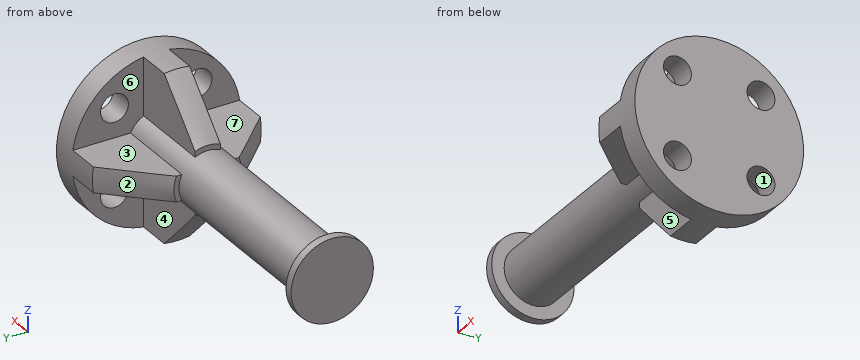
Solid Edge part; units mm, degrees
sketch "Sketch1" plane through (0, 0, 0) normal (-1, 0, 0) x (0, -1, 0)
  circle A0 centre (0, 0) radius 10
extrude "Protrusion1" add sketch "Sketch1" along normal blind 3
sketch "Sketch2" plane through (-3, 0, 0) normal (-1, 0, 0) x (0, -1, 0)
  circle A0 centre (0, 0) radius 3.4
extrude "Protrusion2" add sketch "Sketch2" along normal blind 34.2
sketch "Sketch3" plane through (-3, 0, 0) normal (-1, 0, 0) x (0, -1, 0)
  line L0 (3.0512, 1.5) -> (9.8869, 1.5)
  arc A0 (9.8869, 1.5) -> (9.8869, -1.5) centre (0, 0) cw
  line L1 (3.0512, -1.5) -> (9.8869, -1.5)
  line L2 (3.0512, 1.5) -> (3.0512, -1.5)
  line L3 (1.5, 3.0512) -> (1.5, 9.8869)
  arc A1 (-1.5, 9.8869) -> (1.5, 9.8869) centre (0, 0) cw
  line L4 (-1.5, 3.0512) -> (-1.5, 9.8869)
  line L5 (-1.5, 3.0512) -> (1.5, 3.0512)
  line L6 (-3.0512, 1.5) -> (-9.8869, 1.5)
  arc A2 (-9.8869, 1.5) -> (-9.8869, -1.5) centre (0, 0) ccw
  line L7 (-9.8869, -1.5) -> (-3.0512, -1.5)
  line L8 (-3.0512, -1.5) -> (-3.0512, 1.5)
  line L9 (-1.5, -3.0512) -> (-1.5, -9.8869)
  arc A3 (-1.5, -9.8869) -> (1.5, -9.8869) centre (0, 0) ccw
  line L10 (1.5, -9.8869) -> (1.5, -3.0512)
  line L11 (1.5, -3.0512) -> (-1.5, -3.0512)
extrude "Protrusion3" add sketch "Sketch3" along normal blind 10
chamfer "Chamfer1" distance 6 angle 45 4 edges at (-13, -10, 0) (-13, 0, 10) (-13, 10, 0) (-13, 0, -10)
sketch "Sketch4" plane through (-3, 5.9983, -5.9983) normal (-1, 0, 0) x (0, -1, 0)
  circle A0 centre (1.0486, 1.0486) radius 1.65
  circle A1 centre (10.9481, 1.0486) radius 1.65
  circle A2 centre (10.9481, 10.9481) radius 1.65
  circle A3 centre (1.0486, 10.9481) radius 1.65
extrude "Cutout1" cut sketch "Sketch4" against normal up to next
sketch "Sketch5" plane through (-37.2, 0, 0) normal (-1, 0, 0) x (0, -1, 0)
  circle A0 centre (0, 0) radius 4.875
extrude "Protrusion4" add sketch "Sketch5" against normal blind 1
Read the model definition and answer for the solid it produces. Units are mm, in the model's axes. Face numbers are marked on the shaded views. A direction names the side the tool comes from. Give positions to 0.01 mm unless a question says otherwise; leave off trailing zeros. Order: outer loops, then holes, each group sorted by start corner. A loop starts at its lowest first (then second) coordinate and runs counter-clockwise, first axis right, second up.
(1) Find section D-D (y = -6). Give the number of separate pieces and of enclosed holes in the cut face, plus the area to 3 significant figures.
(2) Straight lines are drawn through the part: L1, parallel to X at y = -0.25, z = -3.5; L2, parallel to Y at x = -7, z = 5.5; L3, parallel to X at y = -3.5, z = -4. For each, find the intervals that lie inside material, in ascending order.
(3) Find section C-C (x = -12). Give the vertices of the cut face in (y, z).
(4) Find section A-A (z = 0). Give the vertices of the cut face in (x, y) (3 decimals), plus the area to 3 significant figures.
(5) For the marked faces 4, 5, 6 and 7, determine the directions among +Z, -Z, +X, -X, +Y, -Y from which every point of the face is accessible in a straight line to the end or side of a thin tool.
(6) Given pin 1 (2.5 mm diameter, centred on y = -4.5, z = -7.5, fed in from -X); pin 2 (4 mm diameter, centred on y = 8, z = -2.5, fed in from -X); pin 3 (2 mm diameter, centred on x = -8.5, z = 7, fed in from +Y), each flat-ended and moving along its own axis, determine where each tip first touches the part or whether it passes through.
(7) For a pull along Z with two mould halves and no side action, classify the marked faces 1, 2 and 3 as released by +Z, released by -Z, zero draft, split by the parting line, or undercut.
Result sheet:
1. separate pieces: 3
1. enclosed holes: 0
1. area: 56.5 mm2
2. L1: x = -37.2 to -36.2, -13 to 0
2. L2: y = -1.5 to 1.5
2. L3: x = -3 to 0
3. outline: (-4.77, -1.5) - (-3.05, -1.5) arc R3.4 ccw to (-1.5, -3.05) - (-1.5, -4.77) arc R5 ccw to (1.5, -4.77) - (1.5, -3.05) arc R3.4 ccw to (3.05, -1.5) - (4.77, -1.5) arc R5 ccw to (4.77, 1.5) - (3.05, 1.5) arc R3.4 ccw to (1.5, 3.05) - (1.5, 4.77) arc R5 ccw to (-1.5, 4.77) - (-1.5, 3.05) arc R3.4 ccw to (-3.05, 1.5) - (-4.77, 1.5) arc R5 ccw to start
4. outline: (-37.2, -4.875) - (-36.2, -4.875) - (-36.2, -3.4) - (-13, -3.4) - (-13, -4) - (-7, -10) - (0, -10) - (0, 10) - (-7, 10) - (-13, 4) - (-13, 3.4) - (-36.2, 3.4) - (-36.2, 4.875) - (-37.2, 4.875) - close
4. area: 392 mm2
5. face 4: -Z, +Y
5. face 5: -Z, -Y
5. face 6: +Z, +Y
5. face 7: +Z, -Y
6. pin 1: stops at x = -3
6. pin 2: stops at x = -10.56
6. pin 3: stops at y = 1.5
7. face 1: undercut
7. face 2: split by the parting line
7. face 3: released by +Z
